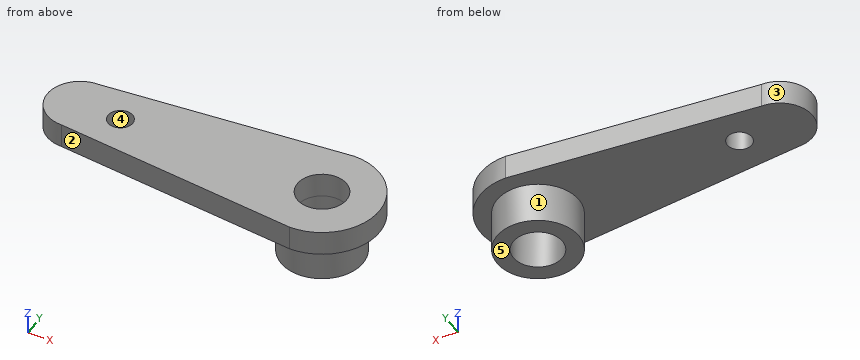
from build123d import *

# Parameters (mm, degrees)
SKETCH1_R           = 5
SKETCH1_R_2         = 3
BOSS_EXTRUDE1_DEPTH = 5
BOSS_EXTRUDE2_DEPTH = 3
SKETCH3_R           = 1.5
CUT_EXTRUDE1_DEPTH  = 3
SKETCH4_R           = 3
CUT_EXTRUDE2_DEPTH  = 3


with BuildPart() as part:
    # Sketch1 → Boss-Extrude1 (new body)
    with BuildSketch(Plane.XY):
        Circle(SKETCH1_R)
        Circle(SKETCH1_R_2, mode=Mode.SUBTRACT)
    extrude(amount=BOSS_EXTRUDE1_DEPTH)

    # Sketch2 → Boss-Extrude2 (add)
    with BuildSketch(Plane.XY.offset(5)):
        with BuildLine():
            Line((-30, 4), (0, 7))
            ThreePointArc((0, 7), (7, 0), (0, -7))
            Line((0, -7), (-30, -4))
            ThreePointArc((-30, -4), (-34, 0), (-30, 4))
        make_face()
    extrude(amount=BOSS_EXTRUDE2_DEPTH)

    # Sketch3 → Cut-Extrude1 (cut)
    with BuildSketch(Plane(origin=(0, 0, 5), x_dir=(-1, 0, 0), z_dir=(0, 0, -1))):
        with Locations((25, 0)):
            Circle(SKETCH3_R)
    extrude(amount=-CUT_EXTRUDE1_DEPTH, mode=Mode.SUBTRACT)

    # Sketch4 → Cut-Extrude2 (cut)
    with BuildSketch(Plane(origin=(0, 0, 5), x_dir=(-1, 0, 0), z_dir=(0, 0, -1))):
        Circle(SKETCH4_R)
    extrude(amount=-CUT_EXTRUDE2_DEPTH, mode=Mode.SUBTRACT)


solid = part.part
Work out the finished part from the listing and answer in its coordinate system (mm). Face numbers are marked on the shaded views. A direction names the side the tool comes from. Give positions to 0.01 mm unless a question says otherwise; leave off trailing zeros. Order: outer loops, then holes, each group sorted by start corner. A loop starts at its lowest first (then second) coordinate and runs counter-clockwise, first axis right, second up. Notation, with made-up numbers: M 12.25,72 L 60.25,72 A14 cw 60.25,79 Z; hole C -3.5,74 d9. An arc over 180 degrees is marked long. Return JSON: item names as keys, results as strings.
Q1. The mould has two halves that part along Y. Classify the marked faces 3, 4 and 5: pulls with the +Y half, pulls with the -Y half, needs draft (parallel to the pull), parting line crosses it, or undercut.
Answer below:
{"face 3": "parting line crosses it", "face 4": "undercut", "face 5": "needs draft"}
Q2. Which of the six approach directions +Z, -Z, +X, -X, +Y, -Y give full straight-line access (tool end or side, diameter ignored) to the marked faces 1 and 2?
Answer below:
{"face 1": "-Z", "face 2": "+Z, -Z, -X, -Y"}
Q3. Find section B-B, the plane z = 6.25. Write down the section's boundary in (x, y), and give its area (3 significant figures).
Answer below:
{"outline": "M -30,-4 L 0,-7 A7 ccw 0,7 L -30,4 A4 ccw Z; hole C -25,0 d3; hole C 0,0 d6", "area": "397 mm^2"}
Q4. Find section A-A, the plane x = -25. Write down the section's boundary in (y, z), and give its area (3 significant figures).
Answer below:
{"outline": "M -4.5,5 L -1.5,5 L -1.5,8 L -4.5,8 Z; M 1.5,5 L 4.5,5 L 4.5,8 L 1.5,8 Z", "area": "18.0 mm^2"}
Q5. Each of these flat-tipped pins is pushed along its axis until it touches: pin 1 (5 mm diameter, centred on x = -25, y = 0, fed in from -Z); pin 2 (4 mm diameter, centred on y = -3, z = 7, fed in from -X). Where does it stop, or does it pass through?
Answer below:
{"pin 1": "stops at z = 5", "pin 2": "stops at x = -33.87"}
Q6. Find section D-D, the plane x = 4. Write down the section's boundary in (y, z).
Answer below:
{"outline": "M -5.74,5 L -3,5 L -3,0 L 3,0 L 3,5 L 5.74,5 L 5.74,8 L -5.74,8 Z"}
Q7. Find section C-C, the plane z = 4.25. Write down the section's boundary in (x, y), and give its area (3 significant figures).
Answer below:
{"outline": "C 0,0 d10; hole C 0,0 d6", "area": "50.3 mm^2"}
Q8. Find the intervals of material crossed by line 1 along X through (y, z) = (1, 5.25); line 2 along Y through (x, z) = (0, 6.75); line 3 along X through (y, z) = (0.75, 7.25), in increasing order. Write a range as [from, to].
Answer below:
{"line 1": "x = [-33.87, -26.12], [-23.88, -2.83], [2.83, 6.93]", "line 2": "y = [-7, -3], [3, 7]", "line 3": "x = [-33.93, -26.3], [-23.7, -2.9], [2.9, 6.96]"}
